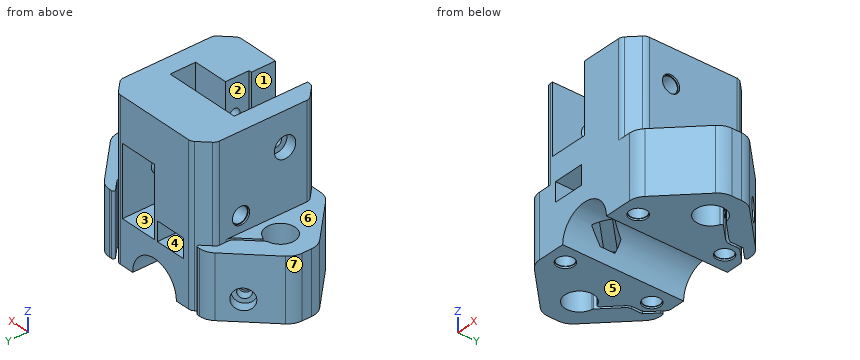
```python
from build123d import *

# Parameters (mm, degrees)
BOSS_EXTRUDE1_DEPTH     = 18
SKETCH2_R               = 7.5
SKETCH2_W               = 9
SKETCH2_H               = 5.5
CUT_EXTRUDE1_DEPTH      = 51.410812332
FILLET1_R               = 5
FILLET2_R               = 0.5
FILLET3_R               = 2
FILLET4_R               = 2.75
CUT_EXTRUDE2_DEPTH      = 15
SKETCH7_R               = 1.6
CUT_EXTRUDE3_DEPTH      = 10
SKETCH8_R               = 2.35
CUT_EXTRUDE4_DEPTH      = 5
SKETCH9_R               = 2.5
CUT_EXTRUDE5_DEPTH      = 0.5
MIRROR3_COPY_1_SKETCH_R = 1.6
MIRROR3_COPY_1_DEPTH    = 10
MIRROR3_COPY_2_SKETCH_R = 2.35
MIRROR3_COPY_2_DEPTH    = 5
MIRROR3_COPY_3_SKETCH_R = 2.5
MIRROR3_COPY_3_DEPTH    = 0.5
BOSS_EXTRUDE2_DEPTH     = 27
SKETCH11_W              = 11
SKETCH11_H              = 20
CUT_EXTRUDE6_DEPTH      = 21.2
SKETCH12_W              = 11
SKETCH12_H              = 3.7
CUT_EXTRUDE7_DEPTH      = 12.5
FILLET5_R               = 10
CUT_EXTRUDE8_REACH      = 67.133
SKETCH13_W              = 11
SKETCH13_H              = 19.8
FILLET6_R               = 10
SKETCH14_W              = 11
SKETCH14_H              = 7.4
CUT_EXTRUDE9_DEPTH      = 12.5
SKETCH15_R              = 2.75
BOSS_EXTRUDE3_DEPTH     = 0.8
BOSS_EXTRUDE3_TAPER     = 30
SKETCH16_W              = 14
SKETCH16_H              = 6.815
CUT_EXTRUDE10_DEPTH     = 0.8
SKETCH19_R              = 2.75
BOSS_EXTRUDE4_DEPTH     = 0.8
BOSS_EXTRUDE4_TAPER     = 30
FILLET7_R               = 2


with BuildPart() as part:
    # Sketch1 → Boss-Extrude1 (new body)
    with BuildSketch(Plane.XY):
        with BuildLine():
            Line((-17.5, 17.5), (-31.5, 3.5))
            Line((-31.5, 3.5), (-31.5, -3.5))
            Line((-31.5, -3.5), (-17.5, -17.5))
            Line((-17.5, -17.5), (17.5, -17.5))
            Line((17.5, -17.5), (31.5, -3.5))
            Line((31.5, -3.5), (31.5, 3.5))
            Line((31.5, 3.5), (17.5, 17.5))
            Line((17.5, 17.5), (13.560660172, 17.5))
            Line((13.560660172, 17.5), (17.25, 13.810660172))
            Line((17.25, 13.810660172), (17.25, 9.845660172))
            Line((17.25, 9.845660172), (22.916347453, 4.179312718))
            ThreePointArc((22.916347453, 4.179312718), (22.602164744, -4.198757241), (21.880882362, 4.154117638))
            Line((21.880882362, 4.154117638), (16.5, 9.535))
            Line((16.5, 9.535), (16.5, 13.5))
            Line((16.5, 13.5), (12.5, 17.5))
            Line((12.5, 17.5), (-12.5, 17.5))
            Line((-12.5, 17.5), (-16.5, 13.5))
            Line((-16.5, 13.5), (-16.5, 9.535))
            Line((-16.5, 9.535), (-21.880882362, 4.154117638))
            ThreePointArc((-21.880882362, 4.154117638), (-22.602164744, -4.198757241), (-22.916347453, 4.179312718))
            Line((-22.916347453, 4.179312718), (-17.25, 9.845660172))
            Line((-17.25, 9.845660172), (-17.25, 13.810660172))
            Line((-17.25, 13.810660172), (-13.560660172, 17.5))
            Line((-13.560660172, 17.5), (-17.5, 17.5))
        make_face()
    extrude(amount=BOSS_EXTRUDE1_DEPTH)

    # Sketch2 → Cut-Extrude1 (cut, through all)
    with BuildSketch(Plane(origin=(0, 17.5, 0), x_dir=(1, 0, 0), z_dir=(0, 1, 0))):
        Circle(SKETCH2_R)
        with Locations((-5.5, -15.25)):
            Rectangle(SKETCH2_W, SKETCH2_H)
    extrude(amount=-CUT_EXTRUDE1_DEPTH, mode=Mode.SUBTRACT)

    # Fillet1
    fillet1_edges = [part.edges().sort_by_distance(p)[0] for p in [
        (17.5, 17.5, 9),
        (31.5, 3.5, 9),
        (31.5, -3.5, 9),
        (17.5, -17.5, 9),
        (-17.5, -17.5, 9),
        (-31.5, -3.5, 9),
        (-31.5, 3.5, 9),
        (-17.5, 17.5, 9),
    ]]
    fillet(fillet1_edges, radius=FILLET1_R)

    # Fillet2
    fillet2_edges = [part.edges().sort_by_distance(p)[0] for p in [
        (-13.560660172, 17.5, 9),
        (-22.916347453, 4.179312718, 9),
        (-21.880882362, 4.154117638, 9),
        (21.880882362, 4.154117638, 9),
        (22.916347453, 4.179312718, 9),
        (13.560660172, 17.5, 9),
    ]]
    fillet(fillet2_edges, radius=FILLET2_R)

    # Fillet3
    fillet3_edges = [part.edges().sort_by_distance(p)[0] for p in [
        (-17.25, 9.845660172, 9),
        (17.25, 9.845660172, 9),
    ]]
    fillet(fillet3_edges, radius=FILLET3_R)

    # Fillet4
    fillet4_edges = [part.edges().sort_by_distance(p)[0] for p in [
        (-16.5, 9.535, 9),
        (16.5, 9.535, 9),
    ]]
    fillet(fillet4_edges, radius=FILLET4_R)

    # Sketch4 → Cut-Revolve1 (revolve, cut)
    with BuildSketch(Plane(origin=(0, 0, 6), x_dir=(-1, 0, 0), z_dir=(0, 0, -1))):
        Polygon((23.439696962, 11.560303038), (25.561017306, 9.438982694), (23.439696962, 7.317662351), (22.555813485, 8.201545827), (14.070532111, -0.283735547), (12.833095244, 0.95370132), align=None)
    cut_revolve1 = revolve(axis=Axis((-23.439696962, 11.560303038, 6), (0.7071067811865471, -0.707106781186548, 0)), mode=Mode.SUBTRACT)

    # Sketch6 → Cut-Extrude2 (cut)
    with BuildSketch(Plane(origin=(-6.893398282, 6.893398282, 0), x_dir=(0, 0, 1), z_dir=(-0.7071067811865471, 0.707106781186548, 0))):
        Polygon((3.425, -9.886676943), (6, -11.373353886), (8.575, -9.886676943), (8.575, -6.913323057), (6, -5.426646114), (3.425, -6.913323057), align=None)
    cut_extrude2 = extrude(amount=-CUT_EXTRUDE2_DEPTH, mode=Mode.SUBTRACT)

    # Mirror1: Cut-Revolve1, Cut-Extrude2 across plane
    add(cut_revolve1.mirror(Plane(origin=(0, 0, 0), x_dir=(0, 0, 1), z_dir=(1, 0, 0))), mode=Mode.SUBTRACT)
    add(cut_extrude2.mirror(Plane(origin=(0, 0, 0), x_dir=(0, 0, 1), z_dir=(1, 0, 0))), mode=Mode.SUBTRACT)

    # Sketch7 → Cut-Extrude3 (cut)
    with BuildSketch(Plane(origin=(0, 0, 0), x_dir=(-1, 0, 0), z_dir=(0, 0, -1))):
        with Locations((-12.5, 12.5)):
            Circle(SKETCH7_R)
    cut_extrude3 = extrude(amount=-CUT_EXTRUDE3_DEPTH, mode=Mode.SUBTRACT)

    # Sketch8 → Cut-Extrude4 (cut)
    with BuildSketch(Plane(origin=(0, 0, 0), x_dir=(-1, 0, 0), z_dir=(0, 0, -1))):
        with Locations((-12.5, 12.5)):
            Circle(SKETCH8_R)
    cut_extrude4 = extrude(amount=-CUT_EXTRUDE4_DEPTH, mode=Mode.SUBTRACT)

    # Sketch9 → Cut-Extrude5 (cut)
    with BuildSketch(Plane(origin=(0, 0, 0), x_dir=(-1, 0, 0), z_dir=(0, 0, -1))):
        with Locations((-12.5, 12.5)):
            Circle(SKETCH9_R)
    cut_extrude5 = extrude(amount=-CUT_EXTRUDE5_DEPTH, mode=Mode.SUBTRACT)

    # Mirror2: Cut-Extrude3, Cut-Extrude4, Cut-Extrude5 across plane
    add(cut_extrude3.mirror(Plane.ZX), mode=Mode.SUBTRACT)
    add(cut_extrude4.mirror(Plane.ZX), mode=Mode.SUBTRACT)
    add(cut_extrude5.mirror(Plane.ZX), mode=Mode.SUBTRACT)

    # Mirror3: Cut-Extrude3, Cut-Extrude4, Cut-Extrude5 across plane
    add(cut_extrude3.mirror(Plane(origin=(0, 0, 0), x_dir=(0, 0, 1), z_dir=(1, 0, 0))), mode=Mode.SUBTRACT)
    add(cut_extrude4.mirror(Plane(origin=(0, 0, 0), x_dir=(0, 0, 1), z_dir=(1, 0, 0))), mode=Mode.SUBTRACT)
    add(cut_extrude5.mirror(Plane(origin=(0, 0, 0), x_dir=(0, 0, 1), z_dir=(1, 0, 0))), mode=Mode.SUBTRACT)

    # Mirror3 copy 1 sketch → Mirror3 copy 1 (cut)
    with BuildSketch(Plane(origin=(0, 0, 0), x_dir=(1, 0, 0), z_dir=(0, 0, -1))):
        with Locations((-12.5, 12.5)):
            Circle(MIRROR3_COPY_1_SKETCH_R)
    extrude(amount=-MIRROR3_COPY_1_DEPTH, mode=Mode.SUBTRACT)

    # Mirror3 copy 2 sketch → Mirror3 copy 2 (cut)
    with BuildSketch(Plane(origin=(0, 0, 0), x_dir=(1, 0, 0), z_dir=(0, 0, -1))):
        with Locations((-12.5, 12.5)):
            Circle(MIRROR3_COPY_2_SKETCH_R)
    extrude(amount=-MIRROR3_COPY_2_DEPTH, mode=Mode.SUBTRACT)

    # Mirror3 copy 3 sketch → Mirror3 copy 3 (cut)
    with BuildSketch(Plane(origin=(0, 0, 0), x_dir=(1, 0, 0), z_dir=(0, 0, -1))):
        with Locations((-12.5, 12.5)):
            Circle(MIRROR3_COPY_3_SKETCH_R)
    extrude(amount=-MIRROR3_COPY_3_DEPTH, mode=Mode.SUBTRACT)

    # Sketch10 → Boss-Extrude2 (add)
    with BuildSketch(Plane.XY.offset(18)):
        Polygon((12.5, 17.5), (-12.5, 17.5), (-16.5, 13.5), (-16.5, -13.5), (-12.5, -17.5), (12.5, -17.5), (16.5, -13.5), (16.5, 13.5), align=None)
    extrude(amount=BOSS_EXTRUDE2_DEPTH)

    # Sketch11 → Cut-Extrude6 (cut)
    with BuildSketch(Plane(origin=(0, 17.5, 0), x_dir=(1, 0, 0), z_dir=(0, 1, 0))):
        with Locations((5.5, -22.5)):
            Rectangle(SKETCH11_W, SKETCH11_H)
    extrude(amount=-CUT_EXTRUDE6_DEPTH, mode=Mode.SUBTRACT)

    # Sketch12 → Cut-Extrude7 (cut)
    with BuildSketch(Plane(origin=(0, 0, 32.5), x_dir=(-1, 0, 0), z_dir=(0, 0, -1))):
        with Locations((-5.5, 1.85)):
            Rectangle(SKETCH12_W, SKETCH12_H)
        Polygon((-11, -3.7), (0, -3.7), (0, -3.591245546), (0, 0), (-11, 0), align=None)
    extrude(amount=-CUT_EXTRUDE7_DEPTH, mode=Mode.SUBTRACT)

    # Fillet5
    fillet5_edges = [part.edges().sort_by_distance(p)[0] for p in [
        (5.5, -3.7, 12.5),
    ]]
    fillet(fillet5_edges, radius=FILLET5_R)

    # Cut-Extrude8: up to this face of the body (flat: up to its plane)
    cut_extrude8_end = Plane(part.part.faces().sort_by_distance((5.5, 3.7, 38.75))[0])
    # Sketch13 → Cut-Extrude8 (cut, up to the picked face)
    with BuildSketch(Plane.XZ.offset(17.5), mode=Mode.PRIVATE) as cut_extrude8_sk1:
        with Locations((-5.5, 35.1)):
            Rectangle(SKETCH13_W, SKETCH13_H)
    cut_extrude8_tool1 = split(extrude(cut_extrude8_sk1.sketch, amount=-CUT_EXTRUDE8_REACH, mode=Mode.PRIVATE), bisect_by=cut_extrude8_end, keep=Keep.BOTH, mode=Mode.PRIVATE)
    add(cut_extrude8_tool1.solids().sort_by(Axis((-5.5, -17.5, 35.1), (0, 1, 0)))[0], mode=Mode.SUBTRACT)

    # Fillet6
    # the kernel refuses this fillet: 10 mm, written as the material it adds along each edge
    with BuildSketch(Plane(origin=(25, 3.7, 25.2), x_dir=(0, 0, 1), z_dir=(-1, 0, 0))) as fillet6_piece_1_section:
        with BuildLine():
            CenterArc((FILLET6_R, -FILLET6_R), FILLET6_R, 90, 90)
            Line((0, -FILLET6_R), (0, 0))
            Line((0, 0), (FILLET6_R, 0))
        make_face()
    fillet6_piece_1 = extrude(amount=36, mode=Mode.PRIVATE)
    fillet6_piece_1 = split(fillet6_piece_1, bisect_by=Plane(origin=(5.5, 3.588944861, 32.5), z_dir=(0, 0, 1)), keep=Keep.TOP, mode=Mode.PRIVATE)
    fillet6_piece_1 = split(fillet6_piece_1, bisect_by=Plane(origin=(11, 3.588944861, 33.172467691), z_dir=(-1, 0, 0)), keep=Keep.TOP, mode=Mode.PRIVATE)
    add(fillet6_piece_1)
    with BuildSketch(Plane(origin=(0, 3.7, 25.2), x_dir=(0, 0, 1), z_dir=(-1, 0, 0))) as fillet6_piece_2:
        with BuildLine():
            CenterArc((FILLET6_R, -FILLET6_R), FILLET6_R, 90, 90)
            Line((0, -FILLET6_R), (0, 0))
            Line((0, 0), (FILLET6_R, 0))
        make_face()
    extrude(amount=11)

    # Sketch14 → Cut-Extrude9 (cut)
    with BuildSketch(Plane.XY.offset(45)):
        with Locations((5.5, 0)):
            Rectangle(SKETCH14_W, SKETCH14_H)
    extrude(amount=-CUT_EXTRUDE9_DEPTH, mode=Mode.SUBTRACT)

    # Sketch15 → Boss-Extrude3 (add)
    with BuildSketch(Plane(origin=(-11, 0, 0), x_dir=(0, 0, -1), z_dir=(1, 0, 0))):
        with Locations((-35.23, -6.365)):
            Circle(SKETCH15_R)
    extrude(amount=BOSS_EXTRUDE3_DEPTH, taper=BOSS_EXTRUDE3_TAPER)

    # Sketch16 → Cut-Extrude10 (cut)
    with BuildSketch(Plane.ZY):
        with Locations((38, -7.1075)):
            Rectangle(SKETCH16_W, SKETCH16_H)
    extrude(amount=-CUT_EXTRUDE10_DEPTH, mode=Mode.SUBTRACT)

    # Sketch17 → Cut-Revolve2 (revolve, cut)
    with BuildSketch(Plane.XY.offset(35.23)):
        Polygon((-16.5, -6.365), (-16.5, -3.265), (-13.5, -3.265), (-13.5, -4.865), (11.5, -4.865), (11.5, -4.115), (16, -4.115), (16, -3.865), (16.5, -3.865), (16.5, -6.365), align=None)
    revolve(axis=Axis((31.947720378, -6.365, 35.23), (-1, 0, 0)), mode=Mode.SUBTRACT)

    # Sketch19 → Boss-Extrude4 (add)
    with BuildSketch(Plane.ZY.offset(-11)):
        with Locations((22.5, 6.365)):
            Circle(SKETCH19_R)
    boss_extrude4 = extrude(amount=BOSS_EXTRUDE4_DEPTH, taper=BOSS_EXTRUDE4_TAPER)

    # Mirror4: Boss-Extrude4 across plane
    add(boss_extrude4.mirror(Plane(origin=(5.5, 0, 0), x_dir=(0, 0, 1), z_dir=(1, 0, 0))))

    # Sketch20 → Cut-Revolve3 (revolve, cut)
    with BuildSketch(Plane.XY.offset(22.5), mode=Mode.PRIVATE) as cut_revolve3_sk:
        Polygon((16.5, 6.365), (16.5, 9.465), (13.5, 9.465), (13.5, 7.865), (-11.5, 7.865), (-11.5, 8.615), (-16, 8.615), (-16, 8.865), (-16.5, 8.865), (-16.5, 6.365), align=None)
    revolve(cut_revolve3_sk.sketch.rotate(Axis((11, 6.365, 22.5), (-1, 0, 0)), 90), axis=Axis((11, 6.365, 22.5), (-1, 0, 0)), mode=Mode.SUBTRACT)

    # Fillet7
    fillet7_edges = [part.edges().sort_by_distance(p)[0] for p in [
        (16.5, -13.5, 31.5),
        (12.5, -17.5, 31.5),
        (-12.5, -17.5, 31.5),
        (-16.5, -13.5, 31.5),
        (-16.5, 13.5, 22.5),
        (-12.5, 17.5, 22.5),
        (12.5, 17.5, 22.5),
        (16.5, 13.5, 22.5),
    ]]
    fillet(fillet7_edges, radius=FILLET7_R)


solid = part.part
```
Verification items for the finished model (mm, model axes). Face numbers are marked on the shaded views. A direction names the side the tool comes from. Give positions to 0.01 mm unless a question says otherwise; leave off trailing zeros. Order: outer loops, then holes, each group sorted by start corner. A loop starts at its lowest first (then second) coordinate and runs counter-clockwise, first axis right, second up. Notation, with made-up numbers: (-34.5, 59) -> (18.5, 59) arc R21 cw to (18.5, 71) -> close; hole circle Ø8 at (9, -36.75). An arc over 180 degrees is marked (long way). One line per item, written item: value.
(1) Sectioned sample at B-B on z = 41.5. Record the cut outline in (x, y) (3 decimals).
Final values:
outline: (-16.5, -12.672) arc R2 ccw to (-15.914, -14.086) -> (-13.086, -16.914) arc R2 ccw to (-11.672, -17.5) -> (-11, -17.5) -> (-11, 3.7) -> (11, 3.7) -> (11, -3.7) -> (0.8, -3.7) -> (0.8, -10.515) -> (0, -10.515) -> (0, -17.5) -> (11.672, -17.5) arc R2 ccw to (13.086, -16.914) -> (15.914, -14.086) arc R2 ccw to (16.5, -12.672) -> (16.5, 12.672) arc R2 ccw to (15.914, 14.086) -> (13.086, 16.914) arc R2 ccw to (11.672, 17.5) -> (-11.672, 17.5) arc R2 ccw to (-13.086, 16.914) -> (-15.914, 14.086) arc R2 ccw to (-16.5, 12.672) -> close
(2) Sectioned sample at A-A on x = -8.5. Record the cut outline in (y, z) (3 decimals), then the cut area to 3 significant figures.
Final values:
outline: (-17.5, 0) -> (17.5, 0) -> (17.5, 12.5) -> (-17.5, 12.5) -> close; (-17.5, 18) -> (17.5, 18) -> (17.5, 45) -> (3.7, 45) -> (3.7, 35.2) arc R10 cw to (-6.3, 25.2) -> (-17.5, 25.2) -> close; hole (-7.584, 6) -> (-5.482, 3.425) -> (-1.277, 3.425) -> (0.826, 6) -> (-1.277, 8.575) -> (-5.482, 8.575) -> close; hole circle Ø3 at (6.365, 22.5)
area: 945 mm^2
(3) Gauge pin test, flat ends, axial feed: pin 1 (5.5 mm diameter, centred on x = -11.5, y = 12, fed in from -Z); pin 2 (2.5 mm diameter, centred on y = -6, z = 36, fed in from +X); pin 3 (12 mm diameter, centred on x = -23, z = 29, fed in from +Y); pin 4 (1.6 mm diameter, centred on x = -13, y = 12, fed in from -Z). Record the tip position at first contact, or that the pin passes through.
Final values:
pin 1: z = 0
pin 2: x = 11.5
pin 3: through
pin 4: z = 10
(4) Tool access check on the marked faces 1, 2 and 3. Record the directions out of +Z, -Z, +X, -X, +Y, -Y that give a thin tool (end or side, any length) a straight path to the whole face; none if there is none.
Final values:
face 1: +Z, -Y
face 2: +Z
face 3: +Y
(5) Draft check along Z on the marked faces 4, 5, 6 and 7. Enter one of: pulls with the +Z half, pulls with the -Z half, needs draft (parallel to the pull), parting line crosses it, or undercut.
Final values:
face 4: undercut
face 5: pulls with the -Z half
face 6: pulls with the +Z half
face 7: needs draft
(6) Scan lines: line 1 along X through (y, z) = (0, 9.75); line 2 along Z through (x, y) = (-6, 6.5); line 3 along X through (y, z) = (8, 25). Record each from-to range of solid material in increasing order. Write a range as [from, to].
Final values:
line 1: [-31.5, -26.7], [-18.3, 18.3], [26.7, 31.5]
line 2: [4.5, 12.5], [18, 21.01], [23.99, 45]
line 3: [-16.5, 0], [11, 13.5]
